```python
from build123d import *

# Parameters (mm, degrees)
F0_W     = 10
F0_H     = 10
F1_DEPTH = 50
F2_W     = 10
F2_H     = 10
F3_DEPTH = 75
F4_W     = 10
F4_H     = 10
F5_DEPTH = 25
F6_R     = 4.99999


# Not quite as in the source:
# - a fillet or chamfer is up to 0.001 mm smaller than in the source, because OpenCascade refuses the exact size


with BuildPart() as f1:
    # F0 (on Top) → F1 (new body)
    with BuildSketch(Plane.XY):
        with Locations((5, 5)):
            Rectangle(F0_W, F0_H)
    extrude(amount=F1_DEPTH)

    # F2 (on face) → F3 (join)
    with BuildSketch(Plane.YZ.offset(10)):
        with Locations((5, 45)):
            Rectangle(F2_W, F2_H)
    extrude(amount=F3_DEPTH)

    # F4 (on face) → F5 (join)
    with BuildSketch(Plane(origin=(0, 0, 40), x_dir=(1, 0, 0), z_dir=(0, 0, -1))):
        with Locations((80, -5)):
            Rectangle(F4_W, F4_H)
    extrude(amount=F5_DEPTH)

    # F6 (radius 5 in the source; OpenCascade refuses exactly that, so slightly less here)
    f6_edges = [f1.edges().sort_by_distance(p)[0] for p in [
        (10, 0, 20),
        (0, 0, 25),
        (0, 10, 25),
        (10, 10, 20),
        (42.5, 0, 50),
        (42.5, 0, 40),
        (42.5, 10, 40),
        (85, 0, 32.5),
        (80, 0, 15),
        (75, 0, 27.5),
        (5, 0, 0),
        (85, 10, 32.5),
        (75, 10, 27.5),
    ]]
    fillet(f6_edges, radius=F6_R)


solid = f1.part
```
The listing builds one solid part. Answer for the finished solid, in the listing's coordinates (mm). A direction names the side the tool comes from. Give positions to 0.01 mm unless a question says otherwise; leave off trailing zeros. Write each loop counter-clockwise with the first axis right and the second up, starting at its lowest first coordinate (ties: lowest second). Pieces come first, ordered by that corner, then holes. Notation, with made-up numbers: (-35.5, 7) -> (-8.5, 7) arc R15 ccw to (-8.5, 29) -> close; hole circle Ø7 at (-15.75, 78). An arc over 180 degrees is marked (long way). Write item = value, one per line. Start each with the question number.
1) Straight lines are drawn through the part: line 1 along Z through (x, y) = (11.5, 5.25); line 2 along X through (y, z) = (4.5, 17.5); line 3 along X through (y, z) = (6.75, 22.5). For each, find the intervals that lie inside material, in ascending order.
2) The part is cut by section C-C, the plane y = 7.75. Determine the outline of the cut face in (x, z), and give its area (3 significant figures).
3) Each of these flat-tipped pins is pushed along its axis until it touches: pin 1 (1 mm diameter, centred on y = 4, z = 18, fed in from -X); pin 2 (2.5 mm diameter, centred on x = 79.5, y = 6.5, fed in from -Z); pin 3 (6 mm diameter, centred on y = 5.5, z = 8, fed in from +X). Where does it stop, or does it pass through?
4) Determine the mould class of faces 1 (the face through (1, 2, 25)), 2 (the face through (80, 7, 15)), 3 (the face through (76, 2, 30)) for opening direction X: +X half, -X half, draft (parallel to the pull), parting line (faces both ways), or undercut.
5) Which of the six approach directions +Z, -Z, +X, -X, +Y, -Y give full straight-line access (tool end or side, diameter ignored) to faces 4 (the face through (80, 2, 16)), 5 (the face through (5, 2, 1)), 6 (the face through (42, 7, 50)), 7 (the face through (43, 8, 41)), 8 (the face through (43, 2, 41))?
Solutions:
q1.line_1 = 40.01 to 50
q1.line_2 = 0.03 to 9.97, 75.03 to 84.97
q1.line_3 = 0.32 to 9.68, 75.32 to 84.68
q2.outline = (0.82, 0) -> (9.18, 0) -> (9.18, 40.82) -> (75.82, 40.82) -> (75.82, 15) -> (84.18, 15) -> (84.18, 50) -> (0.82, 50) -> close
q2.area = 1,320 mm²
q3.pin_1 = 0.03
q3.pin_2 = 15
q3.pin_3 = 10
q4.face_1 = -X half
q4.face_2 = draft
q4.face_3 = undercut
q5.face_4 = -Z, +X, -Y
q5.face_5 = -Z, +X, -X, -Y
q5.face_6 = +Z, +X, -X, +Y, -Y
q5.face_7 = -Z, +Y
q5.face_8 = -Z, -Y
